Could you check a few things on this model? Use its own coordinates, in mm. A direction names the side the tool comes from. Give positions to 0.01 mm unless a question says otherwise; leave off trailing zeros. Loops run counter-clockwise (first coordinate to the right, second up) from the corner with the lowest first, then second, coordinate; pieces in that order, holes last. Notation, with made-up numbers: M -39.75,-14.5 L -4.75,-14.5 A7 ccw -4.75,-10.5 Z; hole C -11.75,61.5 d7. An arc over 180 degrees is marked long. Answer in a Markdown table with one row per item. Add a question column.
1. Which directions (+Z, -Z, +X, -X, +Y, -Y) give clear straight access to the entire face, cutting with the end or side of a thin tool? Please do faces 5 (the flat face through (48, 33, -4)), 6 (the flat face through (67, 63, -36)), 7 (the flat face through (91, 0, -36)).
2. If we section it at C-C on y = 31: Count the separate pieces of the cut face and the enclosed holes in it, then the cut area to 3 significant figures.
3. I need wall thicknesses on line 1 along X through (y, z) = (44, -33.5); line 2 along Z through (x, y) = (46.5, 10); line 3 along Z through (x, y) = (128, 57). Which ranges of each line are inside material? Lowest first, please. Write a range as from..to.
4. If we section it at D-D on x = 42.5: List the corners of the cut face in (y, z) for me.
5. If we section it at A-A on x = 23: List the corners of the cut face in (y, z) for me.
6. If we section it at B-B on z = -25: List the corners of the cut face in (x, y) for me.
7. Thinking about a two-plate mould opening in Z: for faces 1 (the flat face through (67, 34, 0)), 2 (the flat face through (41, 33, -4)), 3 (the flat face through (47, 41, -38)), 4 (the flat face through (83.35, 31, -36)), which applies, released by +Z, released by -Z, zero draft, split by the parting line, or undercut?
8. I'm going to push a flat-ended pin straight in: pin 1 Ø2 at (x, y) = (100.5, 49) entering from -Z. Where does the tip first touch, or does it pass through?
```python
from build123d import *

# Parameters (mm, degrees)
SKETCH_1_W          = 135
SKETCH_1_H          = 38
EXTRUDE_312_DEPTH   = 68
SKETCH_2_W          = 39
SKETCH_2_H          = 15
CUT_EXTRUDE_1_DEPTH = 66
SKETCH_4_W          = 53
SKETCH_4_H          = 9.428155193
CUT_EXTRUDE_2_DEPTH = 66
SKETCH_6_W          = 53
SKETCH_6_H          = 10.153175229
CUT_EXTRUDE_3_DEPTH = 66
SKETCH_7_W          = 30.334064535
SKETCH_7_H          = 3
SKETCH_7_W_2        = 33.750062794
SKETCH_7_W_3        = 31.017264187
CUT_EXTRUDE_4_DEPTH = 66
SKETCH_11_W         = 28.831025302
SKETCH_11_H         = 3.4
SKETCH_11_W_2       = 31.973743699
SKETCH_11_H_2       = 1.4
SKETCH_11_W_3       = 29.240945093
CUT_EXTRUDE_6_DEPTH = 63
SKETCH_12_W         = 31.973743699
SKETCH_12_H         = 2
CUT_EXTRUDE_7_DEPTH = 63


with BuildPart() as part:
    # Эскиз1 → Extrude 312 (new body)
    with BuildSketch(Plane(origin=(0, 0, 0), x_dir=(1, 0, 0), z_dir=(0, 1, 0))):
        with Locations((67.5, 19)):
            Rectangle(SKETCH_1_W, SKETCH_1_H)
    extrude(amount=EXTRUDE_312_DEPTH)

    # Эскиз2 → Вырез-Вытянуть1 (cut)
    with BuildSketch(Plane.XZ):
        with Locations((21.5, -9.1)):
            Rectangle(SKETCH_2_W, SKETCH_2_H)
        with Locations((67.5, -9.1)):
            Rectangle(SKETCH_2_W, SKETCH_2_H)
        with Locations((113.5, -9.1)):
            Rectangle(SKETCH_2_W, SKETCH_2_H)
        with Locations((67.5, -27.1)):
            Rectangle(SKETCH_2_W, SKETCH_2_H)
        with Locations((113.5, -27.1)):
            Rectangle(SKETCH_2_W, SKETCH_2_H)
        with Locations((21.5, -27.1)):
            Rectangle(SKETCH_2_W, SKETCH_2_H)
    extrude(amount=-CUT_EXTRUDE_1_DEPTH, mode=Mode.SUBTRACT)

    # Эскиз4 → Вырез-Вытянуть2 (cut)
    with BuildSketch(Plane.XZ):
        with Locations((67.5, -10.503524842)):
            Rectangle(SKETCH_4_W, SKETCH_4_H)
    extrude(amount=-CUT_EXTRUDE_2_DEPTH, mode=Mode.SUBTRACT)

    # Эскиз6 → Вырез-Вытянуть3 (cut)
    with BuildSketch(Plane.XZ):
        with Locations((67.5, -28.288326327)):
            Rectangle(SKETCH_6_W, SKETCH_6_H)
    extrude(amount=-CUT_EXTRUDE_3_DEPTH, mode=Mode.SUBTRACT)

    # Эскиз7 → Вырез-Вытянуть4 (cut)
    with BuildSketch(Plane.XZ):
        with Locations((22.818742778, -18.1)):
            Rectangle(SKETCH_7_W, SKETCH_7_H)
        with Locations((67.158400174, -18.1)):
            Rectangle(SKETCH_7_W_2, SKETCH_7_H)
        with Locations((112.112937257, -18.1)):
            Rectangle(SKETCH_7_W_3, SKETCH_7_H)
    extrude(amount=-CUT_EXTRUDE_4_DEPTH, mode=Mode.SUBTRACT)

    # Эскиз11 → Вырез-Вытянуть6 (cut)
    with BuildSketch(Plane.XZ):
        with Locations((22.203863092, -36.3)):
            Rectangle(SKETCH_11_W, SKETCH_11_H)
        with Locations((67.36336007, -37.3)):
            Rectangle(SKETCH_11_W_2, SKETCH_11_H_2)
        with Locations((112.591177012, -36.3)):
            Rectangle(SKETCH_11_W_3, SKETCH_11_H)
    extrude(amount=-CUT_EXTRUDE_6_DEPTH, mode=Mode.SUBTRACT)

    # Эскиз12 → Вырез-Вытянуть7 (cut)
    with BuildSketch(Plane.XZ):
        with Locations((67.36336007, -35.6)):
            Rectangle(SKETCH_12_W, SKETCH_12_H)
    extrude(amount=-CUT_EXTRUDE_7_DEPTH, mode=Mode.SUBTRACT)


solid = part.part
```
Results:
| question | item | result |
|---|---|---|
| 1 | face 5 | -Y |
| 1 | face 6 | -Z, -Y |
| 1 | face 7 | +Z, -Z, +X, -X, -Y |
| 2 | separate pieces | 5 |
| 2 | enclosed holes | 0 |
| 2 | area | 754 mm2 |
| 3 | line 1 | 0..2, 41..48, 87..94, 133..135 |
| 3 | line 2 | -38..-33.36, -23.21..-15.22, -5.79..0 |
| 3 | line 3 | -38..-34.6, -19.6..-16.6, -1.6..0 |
| 4 | outline | M 0,-38 L 68,-38 L 68,0 L 0,0 L 0,-5.79 L 66,-5.79 L 66,-15.22 L 0,-15.22 L 0,-23.21 L 66,-23.21 L 66,-33.36 L 0,-33.36 Z |
| 5 | outline | M 0,-1.6 L 66,-1.6 L 66,-34.6 L 63,-34.6 L 63,-38 L 68,-38 L 68,0 L 0,0 Z |
| 6 | outline | M 0,0 L 2,0 L 2,66 L 133,66 L 133,0 L 135,0 L 135,68 L 0,68 Z |
| 7 | face 1 | released by +Z |
| 7 | face 2 | undercut |
| 7 | face 3 | released by -Z |
| 7 | face 4 | zero draft |
| 8 | pin 1 | z = -1.6 |
